The listing builds one solid part. Answer for the finished solid, in the listing's coordinates (mm). A direction names the side the tool comes from. Round coordinates to 2 decimals unless told otherwise and drop trailing zeros. Write each loop counter-clockwise with the first axis right and the second up, starting at its lowest first coordinate (ties: lowest second). Pieces come first, ordered by that corner, then holes. Notation, with made-up numbers: M 14,-14.75 L 63,-14.75 A9 ccw 63,-4.75 Z; hole C 58,-37.5 d10. An arc over 180 degrees is marked long. Write each question's results on one line, items separated by ' | '.
from build123d import *

# Parameters (mm, degrees)
F0_W      = 17
F0_H      = 11
F1_DEPTH  = 18
F3_DEPTH  = 25
F4_W      = 8
F4_H      = 5
F5_DEPTH  = 25
F7_DEPTH  = 25
F8_W      = 6
F8_H      = 3.5
F9_DEPTH  = 17
F10_W     = 6
F10_H     = 3.5
F11_DEPTH = 17


with BuildPart() as f1:
    # F0 (on Front) → F1 (new body)
    with BuildSketch(Plane.XZ):
        with Locations((8.5, 5.5)):
            Rectangle(F0_W, F0_H)
    extrude(amount=F1_DEPTH)

    # F2 (on face) → F3 (cut)
    with BuildSketch(Plane.XZ.offset(18)):
        Polygon((10.5, 9), (10.5, 11), (6.5, 11), (6.5, 9), (8.5, 1), align=None)
    extrude(amount=-F3_DEPTH, mode=Mode.SUBTRACT)

    # F4 (on face) → F5 (cut)
    with BuildSketch(Plane.YZ.offset(17)):
        with Locations((-9, 8.5)):
            Rectangle(F4_W, F4_H)
    extrude(amount=-F5_DEPTH, mode=Mode.SUBTRACT)

    # F6 (on face) → F7 (cut)
    with BuildSketch(Plane.YZ.offset(17)):
        Polygon((-6, 4), (-9, 4), (-12, 4), (-12, 0), (-6, 0), align=None)
    extrude(amount=-F7_DEPTH, mode=Mode.SUBTRACT)

    # F8 (on face) → F9 (join)
    with BuildSketch(Plane.YZ.offset(17)):
        with Locations((-3, -1.75)):
            Rectangle(F8_W, F8_H)
    extrude(amount=-F9_DEPTH)

    # F10 (on face) → F11 (join)
    with BuildSketch(Plane.YZ.offset(17)):
        with Locations((-15, -1.75)):
            Rectangle(F10_W, F10_H)
    extrude(amount=-F11_DEPTH)


solid = f1.part
1) Find the intervals of material crossed by line 1 (Y direction, x = 14.5, z = 6.25); line 2 (Y direction, x = 6.5, z = 3); line 3 (Z direction, x = 3.25, y = -5.5), in increasing order.
Return value:
line 1: -18 to -13, -5 to 0 | line 2: -18 to -12, -6 to 0 | line 3: -3.5 to 6
2) Section A-A (z = 5) is taken. Determine the outline of the cut face in (x, y).
Return value:
outline: M 0,-18 L 7.5,-18 L 7.5,0 L 0,0 Z; M 9.5,-18 L 17,-18 L 17,0 L 9.5,0 Z
3) The mould has two halves that part along Y. Classify faces 6 (the face through (11, 0, 4)), 7 (the face through (13, -5, 8)), 8 (the face through (14, -15, 11)): +Y half, -Y half, draft (parallel to the pull), parting line (faces both ways), or undercut.
Return value:
face 6: +Y half | face 7: undercut | face 8: draft
4) Each of these flat-tipped pins is pushed along its axis until it touches: pin 1 (1.5 mm diameter, centred on y = -4.5, z = 5, fed in from -X); pin 2 (3 mm diameter, centred on x = 12, y = -9, fed in from -Z); pin 3 (2 mm diameter, centred on x = 3, y = -10, fed in from +Z). Where does it stop, or does it pass through?
Return value:
pin 1: x = 0 | pin 2: z = 4 | pin 3: z = 6
5) Section D-D (z = 3.5) is taken. Determine the outline of the cut face in (x, y) (3 decimals), then the cut area to 3 significant figures.
Return value:
outline: M 0,-18 L 7.875,-18 L 7.875,-12 L 0,-12 Z; M 0,-6 L 7.875,-6 L 7.875,0 L 0,0 Z; M 9.125,-18 L 17,-18 L 17,-12 L 9.125,-12 Z; M 9.125,-6 L 17,-6 L 17,0 L 9.125,0 Z | area: 189 mm²
6) A tool of negligible diameter and unlimited length cuts with its end or side. For faces 1 (the face through (13, -9, 4)), 2 (the face through (0, -9, 5)), 3 (the face through (11, -18, 4)), 4 (the face through (10.5, -3, 10)), 5 (the face through (13, -9, 6)), from which of +Z, -Z, +X, -X, +Y, -Y can it reach the whole face along a straight path? Write none if from no direction.
Return value:
face 1: -Z, +X, -X | face 2: +Z, -Z, -X, +Y, -Y | face 3: +Z, -Z, +X, -X, -Y | face 4: +Z, +Y, -Y | face 5: +Z, +X, -X
7) Section C-C (x = 10.25) is taken. Determine the outline of the cut face in (y, z).
Return value:
outline: M -18,-3.5 L -12,-3.5 L -12,4 L -6,4 L -6,-3.5 L 0,-3.5 L 0,8 L -5,8 L -5,6 L -13,6 L -13,8 L -18,8 Z
8) Section B-B (y = -9) is taken. Determine the outline of the cut face in (x, z).
Return value:
outline: M 0,4 L 7.75,4 L 7.25,6 L 0,6 Z; M 9.25,4 L 17,4 L 17,6 L 9.75,6 Z
